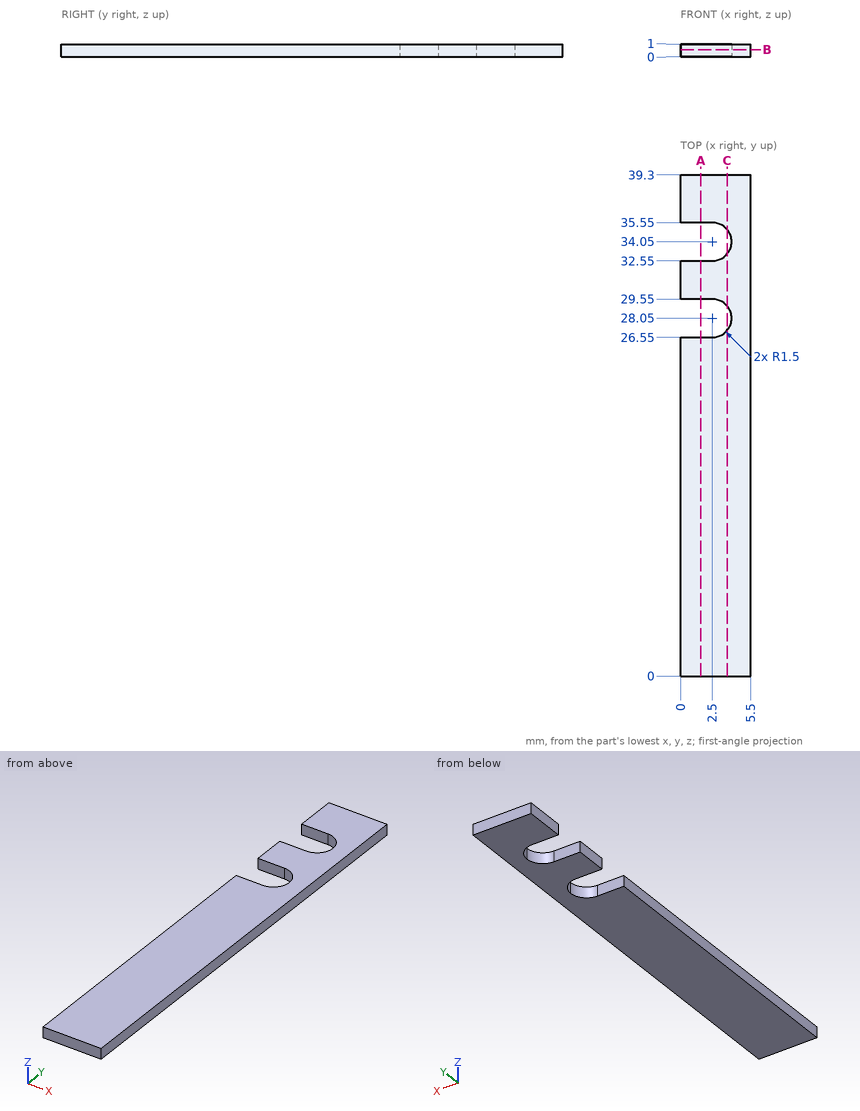
For this review, use the dimensioned drawing (mm, ordinates from the lowest corner) and the shaded views. Round coordinates to 2 decimals unless told otherwise and drop trailing zeros. Order: outer loops, then holes, each group sorted by start corner. A loop starts at its lowest first (then second) coordinate and runs counter-clockwise, first axis right, second up. Notation, with made-up numbers: (15.25, 47.5) -> (57.25, 47.5) arc R26 ccw to (57.25, 85.5) -> close; hole circle Ø3 at (25.25, 60.5). An arc over 180 degrees is marked (long way). Put each result on its own line as item: value.
Q1. Add section A-A on x = 1.6. Write out the cut boundary in (y, z).
Check result:
outline: (0, 0) -> (26.55, 0) -> (26.55, 1) -> (0, 1) -> close; (29.55, 0) -> (32.55, 0) -> (32.55, 1) -> (29.55, 1) -> close; (35.55, 0) -> (39.3, 0) -> (39.3, 1) -> (35.55, 1) -> close
Q2. Insertion check: pin 1 Ø1.5 at (x, y) = (1.5, 4.5) entering from -Z. The pin has a flat end and moves straight along its axis. Give the tip position at first contact, or say it passes through.
Check result:
pin 1: z = 0
Q3. Add section B-B on z = 0.55. Write out the cut boundary in (x, y), plus the area to 3 significant figures.
Check result:
outline: (0, 0) -> (5.5, 0) -> (5.5, 39.3) -> (0, 39.3) -> (0, 35.55) -> (2.5, 35.55) arc R1.5 cw to (2.5, 32.55) -> (0, 32.55) -> (0, 29.55) -> (2.5, 29.55) arc R1.5 cw to (2.5, 26.55) -> (0, 26.55) -> close
area: 194 mm2
Q4. Add section C-C on x = 3.65. Write out the cut boundary in (y, z), plus the area to 3 significant figures.
Check result:
outline: (0, 0) -> (27.09, 0) -> (27.09, 1) -> (0, 1) -> close; (29.01, 0) -> (33.09, 0) -> (33.09, 1) -> (29.01, 1) -> close; (35.01, 0) -> (39.3, 0) -> (39.3, 1) -> (35.01, 1) -> close
area: 35.4 mm2
Q5. For probe 1 along Y at (x, z) = (0.4, 0.95); probe 2 along X at (y, z) = (28, 0.65); probe 3 along X at (y, z) = (35, 0.2), list the stretches that pass through material, from the lowest coordinate up. Write a range as [from, to].
Check result:
probe 1: [0, 26.55], [29.55, 32.55], [35.55, 39.3]
probe 2: [4, 5.5]
probe 3: [3.66, 5.5]
